Check sheet for the modelled part. Datum: model origin and axes. Units: mm. A direction names the side the tool comes from. Round coordinates to 2 decimals unless told otherwise and drop trailing zeros. Order: outer loops, then holes, each group sorted by start corner. A loop starts at its lowest first (then second) coordinate and runs counter-clockwise, first axis right, second up. Notation, with made-up numbers: M -26.75,-35 L -2.75,-35 A12 ccw -2.75,-26 Z; hole C 55,-16 d11. An arc over 180 degrees is marked long. One line per item, written item: value. Start each with the question number.
(1) Thickness scan on L1, parallel to Y at x = 0, z = 9.75 (3 decimals); L2, parallel to Y at x = 2, z = -21; L3, parallel to Y at x = 0, z = -6 (3 decimals). Record the ranges inside material, lowest first.
(2) Depth check by flat-ended pin: pin 1 Ø2 at (x, z) = (-189, -8.5) entering from -Y; pin 2 Ø2 at (x, y) = (6, 101) entering from +Z (3 decimals); pin 3 Ø1.5 at (x, y) = (-35, 40.5) entering from -Z (3 decimals); pin 4 Ø19 at (x, y) = (0, 152.4) entering from +Z. Enter the tip coordinate at first touch or a pass-through.
(3) Cross-section at A-A, the plane y = -50.5. Enter the section's corners in (x, z) (3 decimals), and give its area (3 significant figures).
(4) Cross-section at D-D, the plane y = -21. Enter the section's corners in (x, z) (3 decimals), and give its area (3 significant figures).
(5) Cross-section at C-C, the plane x = -212. Enter the section's corners in (y, z) (3 decimals), and give its area (3 significant figures).
(6) Cross-section at B-B, the plane x = 0. Enter the section's corners in (y, z) (3 decimals), and give its area (3 significant figures).
(7) Release check for a two-part mould opening along X. For faces 6 (the face through (-5.506, -24.796, -0.533)), 7 (the face through (-105.217, -67.362, 0.133)), 8 (the face through (-209, -71, 19.05)) record: released by +X, released by -X, zero draft, split by the parting line, or undercut.
(8) Access from +Z, -Z, +X, -X, +Y, -Y to the whole of each face (thin tool, end or side, straight path). Record for faces 1 (the face through (-209, -71, -19.05)), 2 (the face through (-8.948, -40.293, 24.013)), 3 (the face through (12, 140, -19.05)), 4 (the face through (-61, 8, -9.525)), 5 (the face through (12, 140, 19.05)).
from build123d import *

# Parameters (mm, degrees)
F0_R     = 41.275
F0_R_2   = 25.4
F1_DEPTH = 38.1
F0_R_3   = 15.875
F2_DEPTH = 19.05
F3_DEPTH = 9.525


with BuildPart() as f1:
    # F0 (on Top) → F1 (new body, symmetric)
    with BuildSketch(Plane.XY):
        Circle(F0_R)
        Circle(F0_R_2, mode=Mode.SUBTRACT)
    extrude(amount=F1_DEPTH, both=True)



with BuildPart() as f2:
    # F0 (on Top) → F2 (new body, symmetric)
    with BuildSketch(Plane.XY):
        with BuildLine():
            ThreePointArc((-28.3508788926, 155.971875), (-1.7894497259, 123.8810853173), (28.575, 152.4))
            ThreePointArc((28.575, 152.4), (28.5189146827, 154.1894497259), (28.3508788926, 155.971875))
            ThreePointArc((28.3508788926, 155.971875), (0, 180.975), (-28.3508788926, 155.971875))
        make_face()
        with Locations((0, 152.4)):
            Circle(F0_R_3, mode=Mode.SUBTRACT)
    extrude(amount=F2_DEPTH, both=True)


with BuildPart() as f2b:
    # F0 (on Top) → F2, piece 2 (new body, symmetric)
    with BuildSketch(Plane.XY):
        with BuildLine():
            ThreePointArc((-228.8769827763, -31.7531753778), (-248.6182816065, -65.7437164034), (-215.7407249669, -87.287672125))
            ThreePointArc((-215.7407249669, -87.287672125), (-198.8857315955, -77.4916672845), (-192.2356438897, -59.1660337104))
            ThreePointArc((-192.2356438897, -59.1660337104), (-203.6928900751, -36.285624419), (-228.8769827763, -31.7531753778))
        make_face()
        with Locations((-220.8106438897, -59.1660337104)):
            Circle(F0_R_3, mode=Mode.SUBTRACT)
    extrude(amount=F2_DEPTH, both=True)


with BuildPart() as f1_1:
    add(f1.part)

    add(f2.part)  # F3 merges F2

    add(f2b.part)  # F3 merges F2b
    # F0 (on Top) → F3 (join, symmetric)
    with BuildSketch(Plane.XY):
        with BuildLine():
            ThreePointArc((28.3508788926, 155.971875), (28.5189146827, 154.1894497259), (28.575, 152.4))
            ThreePointArc((28.575, 152.4), (-1.7894497259, 123.8810853173), (-28.3508788926, 155.971875))
            Line((-28.3508788926, 155.971875), (-43.1138110854, 38.7947333871))
            ThreePointArc((-43.1138110854, 38.7947333871), (-48.9692257639, 25.5101831903), (-61.144513313, 17.6027482025))
            Line((-61.144513313, 17.6027482025), (-228.8769827763, -31.7531753778))
            ThreePointArc((-228.8769827763, -31.7531753778), (-203.6928900751, -36.285624419), (-192.2356438897, -59.1660337104))
            ThreePointArc((-192.2356438897, -59.1660337104), (-198.8857315955, -77.4916672845), (-215.7407249669, -87.287672125))
            Line((-215.7407249669, -87.287672125), (8.4456997402, -46.8701480785))
            ThreePointArc((8.4456997402, -46.8701480785), (38.3812204043, -28.1961441562), (47.251464821, 5.953125))
            Line((47.251464821, 5.953125), (28.3508788926, 155.971875))
        make_face()
        Circle(F0_R, mode=Mode.SUBTRACT)
    extrude(amount=F3_DEPTH, both=True)


solid = f1_1.part
Values found:
1. L1: -41.275 to -25.4, 25.4 to 41.275, 123.825 to 136.525, 168.275 to 180.975
1. L2: -41.23 to -25.32, 25.32 to 41.23
1. L3: -48.393 to -25.4, 25.4 to 136.525, 168.275 to 180.975
2. pin 1: y = -82.65
2. pin 2: z = 9.525
2. pin 3: z = -9.525
2. pin 4: through
3. outline: M -248.04,-19.05 L -234.112,-19.05 L -234.112,19.05 L -248.04,19.05 Z; M -207.51,-19.05 L -193.581,-19.05 L -193.581,-9.525 L -11.688,-9.525 L -11.688,9.525 L -193.581,9.525 L -193.581,19.05 L -207.51,19.05 Z
3. area: 4,530 mm^2
4. outline: M -192.333,-9.525 L -35.533,-9.525 L -35.533,-38.1 L -14.288,-38.1 L -14.288,38.1 L -35.533,38.1 L -35.533,9.525 L -192.333,9.525 Z; M 14.288,-38.1 L 35.533,-38.1 L 35.533,-9.525 L 42.745,-9.525 L 42.745,9.525 L 35.533,9.525 L 35.533,38.1 L 14.288,38.1 Z
4. area: 6,360 mm^2
5. outline: M -86.613,-9.525 L -86.349,-9.525 L -86.349,-19.05 L -72.372,-19.05 L -72.372,19.05 L -86.349,19.05 L -86.349,9.525 L -86.613,9.525 Z; M -45.96,-19.05 L -31.983,-19.05 L -31.983,-9.525 L -26.787,-9.525 L -26.787,9.525 L -31.983,9.525 L -31.983,19.05 L -45.96,19.05 Z
5. area: 1,170 mm^2
6. outline: M -48.393,-9.525 L -41.275,-9.525 L -41.275,-38.1 L -25.4,-38.1 L -25.4,38.1 L -41.275,38.1 L -41.275,9.525 L -48.393,9.525 Z; M 25.4,-38.1 L 41.275,-38.1 L 41.275,-9.525 L 123.825,-9.525 L 123.825,-19.05 L 136.525,-19.05 L 136.525,19.05 L 123.825,19.05 L 123.825,9.525 L 41.275,9.525 L 41.275,38.1 L 25.4,38.1 Z; M 168.275,-19.05 L 180.975,-19.05 L 180.975,19.05 L 168.275,19.05 Z
6. area: 5,100 mm^2
7. face 6: undercut
7. face 7: released by +X
7. face 8: zero draft
8. face 1: -Z, -X, +Y, -Y
8. face 2: +Z
8. face 3: -Z, +X, -X, +Y
8. face 4: -Z
8. face 5: +Z, +X, -X, +Y
